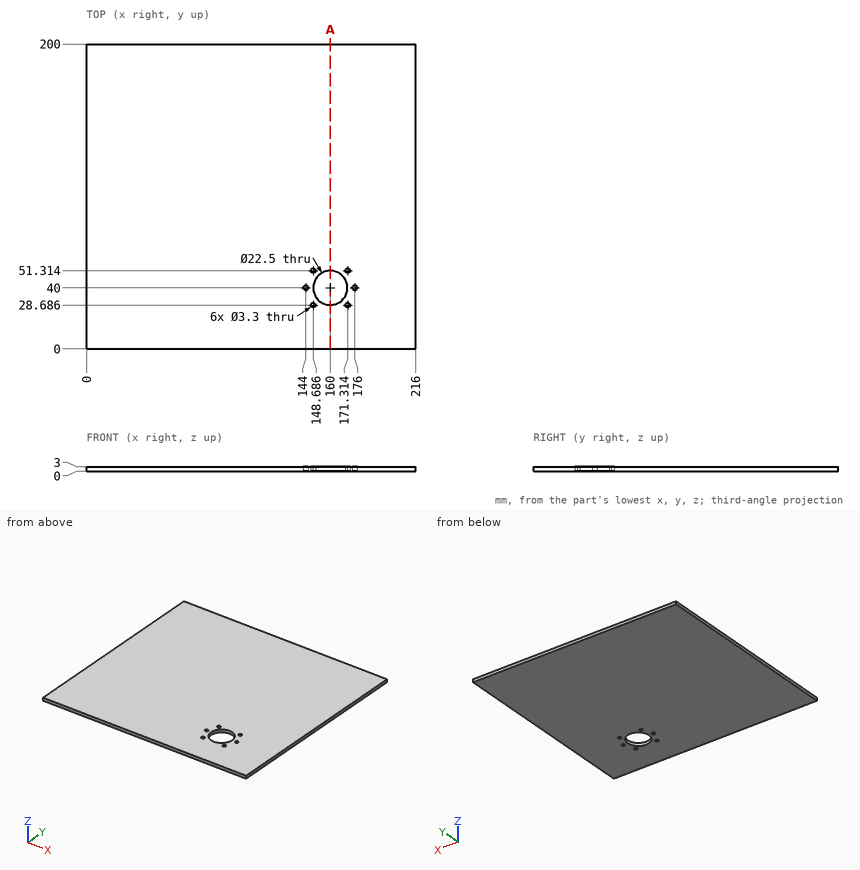
Answer from the drawing. Dimensions are ordinates in mm from the lowest x, y and z of the part. Round coordinates to 2 decimals unless told otherwise and drop trailing zeros. Write each loop counter-clockwise with the first axis right and the second up, starting at its lowest first coordinate (ties: lowest second). Pieces come first, ordered by that corner, then holes. Notation, with made-up numbers: M 1,-11.75 L 27,-11.75 A21 cw 27,13.25 Z; hole C -1,-5 d9. An arc over 180 degrees is marked long. One line per item, written item: value.
Q1. Find section A-A on x = 160. Write down the section's boundary in (y, z).
Data:
outline: M 0,0 L 28.75,0 L 28.75,3 L 0,3 Z; M 51.25,0 L 200,0 L 200,3 L 51.25,3 Z
Q2. Flat-ended cylindrical pins translate along their axes: pin 1 Ø1 at (y, z) = (164, 1.5) entering from -X; pin 2 Ø20 at (x, y) = (160, 40) entering from -Z. Find the tip coordinate at first contact, or state that the pin passes through.
Data:
pin 1: x = 0
pin 2: through
Q3. Straight lines are drawn through the part: line 1 (Y direction, x = 176, z = 1.5); line 2 (Y direction, x = 160, z = 1.2); line 3 (Y direction, x = 147.5, z = 1.25). For each, find the intervals that lie inside material, in ascending order. Write a range as [from, to].
Data:
line 1: [0, 38.35], [41.65, 200]
line 2: [0, 28.75], [51.25, 200]
line 3: [0, 27.54], [29.83, 50.17], [52.46, 200]
